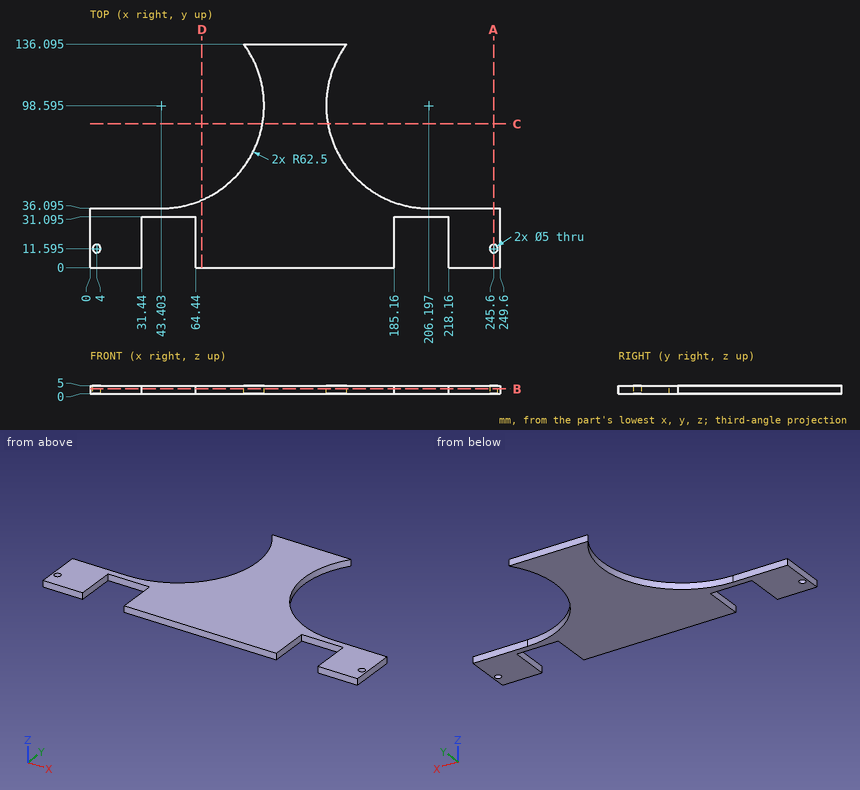
Check sheet for the drawn part. Datum: minimum x, y, z corner. Units: mm. Round coordinates to 2 decimals unless told otherwise and drop trailing zeros. Order: outer loops, then holes, each group sorted by start corner. A loop starts at its lowest first (then second) coordinate and runs counter-clockwise, first axis right, second up.
1) Scan lines: line 1 (X direction, y = 27, z = 2.5); line 2 (Y direction, x = 245.6, z = 1.75) (1 decimal); line 3 (X direction, y = 12.5, z = 4.6). Record each from-to range of solid material in increasing order.
2) Section check B-B (z = 3.1). Record the boundary of the cut face in (x, y) (1 decimal).
3) Go/stop test with flat-tipped pins: pin 1 Ø1 at (x, y) = (142, 122.5) entering from -Z; pin 2 Ø2 at (y, z) = (116, 1) entering from +X; pin 3 Ø1.5 at (x, z) = (197.5, 2.5) entering from -Y (1 decimal). Record where each tip stops, or that it passes through.
4) Section check A-A (x = 245.6). Record the boundary of the cut face in (y, z) (1 decimal).
5) Section check D-D (x = 68). Record the boundary of the cut face in (y, z).
6) Section check C-C (y = 87.5). Record the boundary of the cut face in (x, z).
Result:
1. line 1: x = 0 to 31.44, 64.44 to 185.16, 218.16 to 249.6
1. line 2: y = 0 to 9.1, 14.1 to 36.1
1. line 3: x = 0 to 1.67, 6.33 to 31.44, 64.44 to 185.16, 218.16 to 243.27, 247.93 to 249.6
2. outline: (0, 0) - (31.4, 0) - (31.4, 31.1) - (64.4, 31.1) - (64.4, 0) - (185.2, 0) - (185.2, 31.1) - (218.2, 31.1) - (218.2, 0) - (249.6, 0) - (249.6, 36.1) - (206.2, 36.1) arc R62.5 cw to (156.2, 136.1) - (93.4, 136.1) arc R62.5 cw to (43.4, 36.1) - (0, 36.1) - close; hole circle Ø5 at (4, 11.6); hole circle Ø5 at (245.6, 11.6)
3. pin 1: stops at z = 0
3. pin 2: stops at x = 146.47
3. pin 3: stops at y = 31.1
4. outline: (0, 0) - (9.1, 0) - (9.1, 5) - (0, 5) - close; (14.1, 0) - (36.1, 0) - (36.1, 5) - (14.1, 5) - close
5. outline: (0, 0) - (41.14, 0) - (41.14, 5) - (0, 5) - close
6. outline: (104.91, 0) - (144.69, 0) - (144.69, 5) - (104.91, 5) - close
